```python
from build123d import *

# Parameters (mm, degrees)
BOSS_EXTRUDE1_DEPTH  = 2
CUT_EXTRUDE1_DEPTH   = 7
MIRROR2_COPY_1_DEPTH = 7
SKETCH4_W            = 10
SKETCH4_H            = 30
CUT_EXTRUDE2_DEPTH   = 2
FILLET1_R            = 2


with BuildPart() as part:
    # Sketch2 → Boss-Extrude1 (new, symmetric)
    with BuildSketch(Plane(origin=(0, 0, 0), x_dir=(1, 0, 0), z_dir=(0, 1, 0))):
        Polygon((-25, -8), (-30, -8), (-30, -15), (30, -15), (30, -8), (25, -8), (25, 8), (30, 8), (30, 15), (-30, 15), (-30, 8), (-25, 8), align=None)
    extrude(amount=BOSS_EXTRUDE1_DEPTH, both=True)

    # Sketch3 → Cut-Extrude1 (cut)
    with BuildSketch(Plane(origin=(30, 0, 0), x_dir=(0, 0, -1), z_dir=(1, 0, 0))):
        with BuildLine():
            Line((-12.3, 2), (-12.74567474, 1.335640138))
            ThreePointArc((-12.74567474, 1.335640138), (-11.5, -1), (-10.25432526, 1.335640138))
            Line((-10.25432526, 1.335640138), (-10.7, 2))
            Line((-10.7, 2), (-12.3, 2))
        make_face()
    cut_extrude1 = extrude(amount=-CUT_EXTRUDE1_DEPTH, mode=Mode.SUBTRACT)

    # Mirror1: Cut-Extrude1 across plane
    add(cut_extrude1.mirror(Plane(origin=(0, 0, 0), x_dir=(0, 0, 1), z_dir=(1, 0, 0))), mode=Mode.SUBTRACT)

    # Mirror2: Cut-Extrude1 across plane
    add(cut_extrude1.mirror(Plane.XY), mode=Mode.SUBTRACT)

    # Mirror2 copy 1 sketch → Mirror2 copy 1 (cut)
    with BuildSketch(Plane.ZY.offset(30)):
        with BuildLine():
            Line((-12.3, 2), (-12.74567474, 1.335640138))
            ThreePointArc((-12.74567474, 1.335640138), (-11.5, -1), (-10.25432526, 1.335640138))
            Line((-10.25432526, 1.335640138), (-10.7, 2))
            Line((-10.7, 2), (-12.3, 2))
        make_face()
    extrude(amount=-MIRROR2_COPY_1_DEPTH, mode=Mode.SUBTRACT)

    # Sketch4 → Cut-Extrude2 (cut)
    with BuildSketch(Plane(origin=(0, 2, 0), x_dir=(1, 0, 0), z_dir=(0, 1, 0))):
        Rectangle(SKETCH4_W, SKETCH4_H)
    extrude(amount=-CUT_EXTRUDE2_DEPTH, mode=Mode.SUBTRACT)

    # Fillet1
    fillet1_edges = [part.edges().sort_by_distance(p)[0] for p in [
        (5, 1, -15),
        (5, 1, 15),
        (-5, 1, 15),
        (-5, 1, -15),
        (-25, 0, -8),
        (-30, 0, -8),
        (-30, 0, -15),
        (30, 0, -15),
        (30, 0, -8),
        (25, 0, -8),
        (25, 0, 8),
        (30, 0, 8),
        (30, 0, 15),
        (-30, 0, 15),
        (-30, 0, 8),
        (-25, 0, 8),
    ]]
    fillet(fillet1_edges, radius=FILLET1_R - 0.0001)  # a hair under: the kernel refuses the full size


solid = part.part
```
Verification items for the finished model (mm, model axes). A direction names the side the tool comes from. Give positions to 0.01 mm unless a question says otherwise; leave off trailing zeros. Loops run counter-clockwise (first coordinate to the right, second up) from the corner with the lowest first, then second, coordinate; pieces in that order, holes last. Notation, with made-up numbers: M 24.5,65.5 L 53.5,65.5 A28 cw 53.5,85.5 Z; hole C 81.5,-6.75 d8. An arc over 180 degrees is marked long. One line per question, with ' | ' between items.
Item 1: Draft check along X on faces 1 (the face through (23, 1, 12)), 2 (the face through (5.6, 0.99, -14.43)), 3 (the face through (-30, -1.3, 11.5)). Enter one of: +X half, -X half, draft (parallel to the pull), parting line (faces both ways), or undercut.
Completed:
face 1: +X half | face 2: undercut | face 3: -X half
Item 2: Thickness scan on line 1 (Z direction, x = 28, y = 0.5); line 2 (Z direction, x = -24.5, y = 0.5); line 3 (Z direction, x = -26.5, y = 0.5). Record the ranges inside material, lowest first. Write a range as [from, to].
Completed:
line 1: z = [-15, -13], [-10, -8], [8, 10], [13, 15] | line 2: z = [-15, -13], [-10, 10], [13, 15] | line 3: z = [-15, -13], [-10, -7.94], [7.94, 10], [13, 15]
Item 3: Tool access check on faces 4 (the face through (-25.6, -0.03, 7.43)), 5 (the face through (-23, 1, 12)), 6 (the face through (-5, 1, 0)), 7 (the face through (25.57, 0.03, -7.4)), 8 (the face through (26.5, -1, -11.5)). Record the directions out of +Z, -Z, +X, -X, +Y, -Y that give a thin tool (end or side, any length) a straight path to the whole face; none if there is none.
Completed:
face 4: -X, +Y, -Y | face 5: -X | face 6: +Z, -Z, +Y | face 7: +X, +Y, -Y | face 8: +X
Item 4: Section check D-D, the plane x = -3. Record the cut outline in (y, z), plus the area to 3 significant figures.
Completed:
outline: M -2,-15 L 0,-15 L 0,15 L -2,15 Z | area: 60.0 mm^2
Item 5: Section check C-C, the plane z = 11.5. Record the cut outline in (x, y).
Completed:
outline: M -30,-2 L 30,-2 L 30,-1 L 23,-1 L 23,2 L 5,2 L 5,0 L -5,0 L -5,2 L -23,2 L -23,-1 L -30,-1 Z
Item 6: Section check A-A, the plane z = 0.5. Record the cut outline in (x, y).
Completed:
outline: M -25,-2 L 25,-2 L 25,2 L 5,2 L 5,0 L -5,0 L -5,2 L -25,2 Z
Item 7: Depth check by flat-ended pin: P1, Ø1.8, axis at y = 0.5, z = -11.5, coming from the -X side; P2, Ø1.5, axis at y = 0, z = 7, coming from the +X side; P3, Ø1, axis at y = -0.5, z = -2.5, coming from the +X side. Enter the tip coordinate at first touch or a pass-through.
Completed:
P1: stops at x = -23 | P2: stops at x = 26.03 | P3: stops at x = 25
Item 8: Section check B-B, the plane x = -26. Record the cut outline in (y, z).
Completed:
outline: M -2,-15 L 2,-15 L 2,-12.3 L 1.34,-12.75 A1.5 cw long 1.34,-10.25 L 2,-10.7 L 2,-7.73 L -2,-7.73 Z; M -2,7.73 L 2,7.73 L 2,10.7 L 1.34,10.25 A1.5 cw long 1.34,12.75 L 2,12.3 L 2,15 L -2,15 Z
